Here's the drawing with two shaded views (mm, measured from the low corner). I have some questions. Coordinates: 2 decimals unless noted, no trailing zeros. Write each loop counter-clockwise with the first axis right and the second up, starting at its lowest first coordinate (ties: lowest second). Pieces come first, ordered by that corner, then holes. Notation, with made-up numbers: M -4,4 L 4,4 A20 cw 4,26 Z; hole C 83.5,34.5 d4. An arc over 180 degrees is marked long. Answer as CSV lines item,"result". Start each with the question number.
Item 1: If I drill on line 1 along Y through (x, z) = (5, 6.75); line 2 along Z through (x, y) = (14.5, 1.9), over which ranges is the centre line in solid material (lowest first)? Write a range as [from, to].
Item 2: Suppose I cut it at A-A, the plane y = 3. Write out the boundary of the cut face in (x, z), and give its area (3 significant figures).
Item 3: I'm going to push flat-ended pins straight in: P1, Ø2, axis at x = 15, y = 3, coming from the -Z side; P2, Ø3, axis at x = 5, y = 3, coming from the +Z side. Where does each tip first touch, or does it pass through?
Item 4: Suppose I cut it at B-B, the plane x = 5. Write out the boundary of the cut face in (y, z).
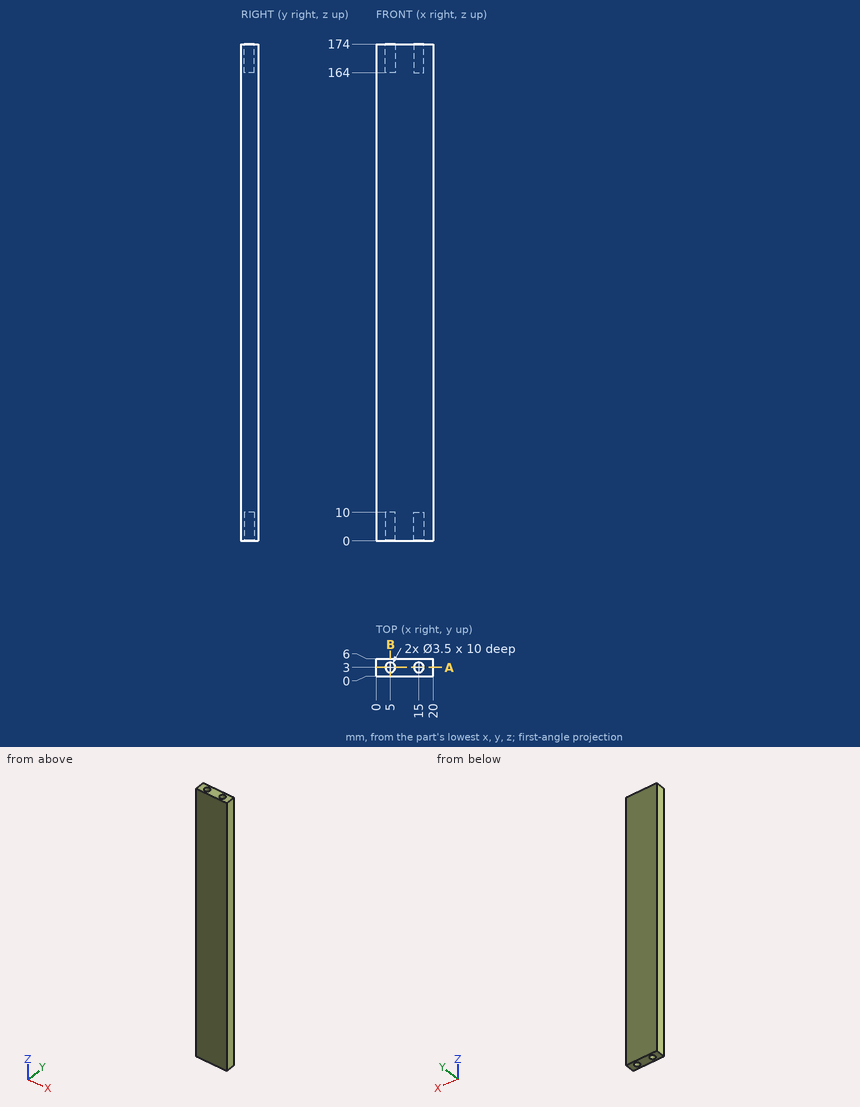
Ans:
1,line 1,"y = [0, 1.25], [4.75, 6]"
1,line 2,"z = [10, 164]"
2,outline,"M 0,0 L 3.25,0 L 3.25,10 L 6.75,10 L 6.75,0 L 13.25,0 L 13.25,10 L 16.75,10 L 16.75,0 L 20,0 L 20,174 L 16.75,174 L 16.75,164 L 13.25,164 L 13.25,174 L 6.75,174 L 6.75,164 L 3.25,164 L 3.25,174 L 0,174 Z"
2,area,"3,340 mm^2"
3,P1,"stops at z = 10"
3,P2,"stops at z = 164"
4,outline,"M 0,0 L 1.25,0 L 1.25,10 L 4.75,10 L 4.75,0 L 6,0 L 6,174 L 4.75,174 L 4.75,164 L 1.25,164 L 1.25,174 L 0,174 Z"
